```python
from build123d import *

# Parameters (mm, degrees)
BOSS_EXTRUDE1_DEPTH                               = 6.35
TAP_DRILL_FOR_6_32_TAP1_D                         = 2.7051
TAP_DRILL_FOR_6_32_TAP1_DEPTH                     = 12.7
TAP_DRILL_FOR_6_32_TAP1_TIP                       = 0.81269403
CSK_FOR_6_FLAT_HEAD_MACHINE_SCREW_100_D           = 3.7973
CSK_FOR_6_FLAT_HEAD_MACHINE_SCREW_100_CSINK_D     = 7.0866
CSK_FOR_6_FLAT_HEAD_MACHINE_SCREW_100_CSINK_ANGLE = 100


with BuildPart() as part:
    # Sketch1 → Boss-Extrude1 (new body)
    with BuildSketch(Plane.XY):
        Polygon((0, 23.8125), (-6.35, 23.8125), (-6.35, 25.4), (-38.1, 25.4), (-38.1, 23.8125), (-31.75, 23.8125), (-31.75, 1.5875), (-38.1, 1.5875), (-38.1, 0), (-6.35, 0), (-6.35, 1.5875), (0, 1.5875), align=None)
    extrude(amount=BOSS_EXTRUDE1_DEPTH)

    # Tap Drill for #6-32 Tap1
    with Locations(Plane.ZY.offset(31.75)):
        with Locations((3.175, 12.7)):
            Hole(TAP_DRILL_FOR_6_32_TAP1_D / 2, depth=TAP_DRILL_FOR_6_32_TAP1_DEPTH)
            with Locations((0, 0, -(TAP_DRILL_FOR_6_32_TAP1_DEPTH + TAP_DRILL_FOR_6_32_TAP1_TIP / 2))):  # 118° drill point
                Cone(0, TAP_DRILL_FOR_6_32_TAP1_D / 2, TAP_DRILL_FOR_6_32_TAP1_TIP, mode=Mode.SUBTRACT)

    # CSK for #6 Flat Head Machine Screw (100)1 (through all)
    with Locations(Plane(origin=(0, 0, 0), x_dir=(-1, 0, 0), z_dir=(0, 0, -1))):
        with Locations((3.175, 12.7)):
            CounterSinkHole(CSK_FOR_6_FLAT_HEAD_MACHINE_SCREW_100_D / 2, CSK_FOR_6_FLAT_HEAD_MACHINE_SCREW_100_CSINK_D / 2, counter_sink_angle=CSK_FOR_6_FLAT_HEAD_MACHINE_SCREW_100_CSINK_ANGLE)


solid = part.part
```
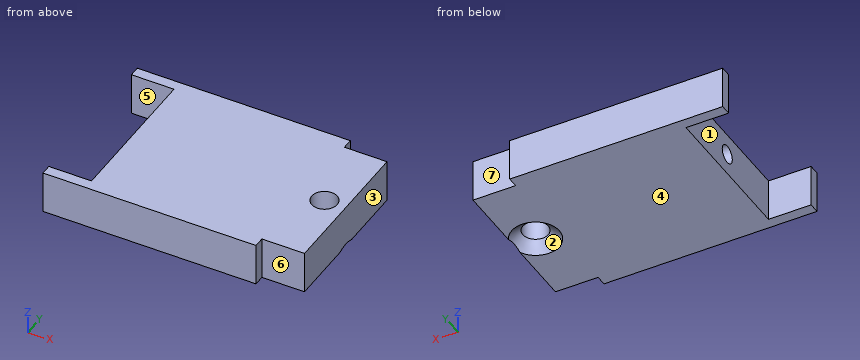
Can you work these out from the model? Positions are in its coordinate system, mm. Face numbers are marked on the shaded views. A direction names the side the tool comes from. Coordinates: 2 decimals unless noted, no trailing zeros. Loops run counter-clockwise (first coordinate to the right, second up) from the corner with the lowest first, then second, coordinate; pieces in that order, holes last. Notation, with made-up numbers: (71.5, 52.5) -> (105.5, 52.5) arc R19 ccw to (105.5, 64.5) -> close; hole circle Ø1 at (-32, 73). An arc over 180 degrees is marked (long way). Answer as a JSON object with one key per item and string values.
1) Imagine slicing it at C-C (y = 22). Please give me the cut outline in (x, z), then the cut area to 3 significant figures.
Results:
{"outline": "(-31.75, 0) -> (0, 0) -> (0, 6.35) -> (-31.75, 6.35) -> close", "area": "202 mm^2"}
2) If I drill on line 1 (X direction, y = 12.7, z = 5.25); line 2 (Z direction, x = -28.5, y = 12.7); line 3 (Y direction, x = -34, z = 6), over which ranges is the centre line in solid material (lowest first)?
Results:
{"line 1": "x = -31.75 to -5.07, -1.28 to 0", "line 2": "z = 0 to 1.82, 4.53 to 6.35", "line 3": "y = 0 to 1.59, 23.81 to 25.4"}
3) Thinking about a two-plate mould opening in X: for the marked faces 1, 2, 3 and 4, which applies, pulls with the +X half, pulls with the -X half, needs draft (parallel to the pull), parting line crosses it, or undercut?
Results:
{"face 1": "pulls with the -X half", "face 2": "undercut", "face 3": "pulls with the +X half", "face 4": "needs draft"}
4) For the marked faces 5, 6 and 7, which set-ups out of +Z, -Z, +X, -X, +Y, -Y let a thin tool reach every point of the face, with its end or its side?
Results:
{"face 5": "+Z, -Z, -X", "face 6": "+Z, -Z, +X, -Y", "face 7": "+Z, -Z, +X, +Y"}
5) For P1, Ø0.5, axis at y = 24.5, z = 3, coming from the +X side; P2, Ø1.5, axis at x = -4, z = 3.5, coming from the -Y side, each with a flat end and sliding along its axis, tell me the tip position at first contact or that it passes through.
Results:
{"P1": "stops at x = -6.35", "P2": "stops at y = 1.59"}
6) Imagine slicing it at A-A (x = -31). Please give me the cut outline in (y, z) (3 decimals).
Results:
{"outline": "(0, 0) -> (25.4, 0) -> (25.4, 6.35) -> (0, 6.35) -> close; hole circle Ø2.705 at (12.7, 3.175)"}
